from build123d import *

# Parameters (mm, degrees)
F0_W     = 274.2
F0_H     = 251.2
F1_DEPTH = 1
F3_DEPTH = 1.001
F4_R     = 1


with BuildPart() as f1:
    # F0 (on Top) → F1 (new body)
    with BuildSketch(Plane.XY):
        Rectangle(F0_W, F0_H)
    extrude(amount=F1_DEPTH)

    # F2 (on face) → F3 (cut, through all)
    with BuildSketch(Plane.XY.offset(1)):
        Polygon((-127.1, -66.8), (-127.1, -115.6), (-104.7, -115.6), (-104.7, -113.6), (-92.7, -113.6), (-92.7, -115.6), (-70.3, -115.6), (-70.3, -6), (-127.1, -6), (-127.1, -54.8), (-125.1, -54.8), (-125.1, -66.8), align=None)
        Polygon((-4.5, -6), (-61.3, -6), (-61.3, -54.8), (-59.3, -54.8), (-59.3, -66.8), (-61.3, -66.8), (-61.3, -115.6), (-38.9, -115.6), (-38.9, -113.6), (-26.9, -113.6), (-26.9, -115.6), (-4.5, -115.6), align=None)
        Polygon((61.3, -6), (4.5, -6), (4.5, -54.8), (6.5, -54.8), (6.5, -66.8), (4.5, -66.8), (4.5, -115.6), (26.9, -115.6), (26.9, -113.6), (38.9, -113.6), (38.9, -115.6), (61.3, -115.6), align=None)
        Polygon((127.1, -6), (70.3, -6), (70.3, -54.8), (72.3, -54.8), (72.3, -66.8), (70.3, -66.8), (70.3, -115.6), (92.7, -115.6), (92.7, -113.6), (104.7, -113.6), (104.7, -115.6), (127.1, -115.6), align=None)
        Polygon((127.1, 115.6), (70.3, 115.6), (70.3, 66.8), (72.3, 66.8), (72.3, 54.8), (70.3, 54.8), (70.3, 6), (92.7, 6), (92.7, 8), (104.7, 8), (104.7, 6), (127.1, 6), align=None)
        Polygon((61.3, 115.6), (4.5, 115.6), (4.5, 66.8), (6.5, 66.8), (6.5, 54.8), (4.5, 54.8), (4.5, 6), (26.9, 6), (26.9, 8), (38.9, 8), (38.9, 6), (61.3, 6), align=None)
        Polygon((-4.5, 115.6), (-61.3, 115.6), (-61.3, 66.8), (-59.3, 66.8), (-59.3, 54.8), (-61.3, 54.8), (-61.3, 6), (-38.9, 6), (-38.9, 8), (-26.9, 8), (-26.9, 6), (-4.5, 6), align=None)
        Polygon((-70.3, 115.6), (-127.1, 115.6), (-127.1, 66.8), (-125.1, 66.8), (-125.1, 54.8), (-127.1, 54.8), (-127.1, 6), (-104.7, 6), (-104.7, 8), (-92.7, 8), (-92.7, 6), (-70.3, 6), align=None)
    extrude(amount=-F3_DEPTH, mode=Mode.SUBTRACT)

    # F4
    f4_edges = [f1.edges().sort_by_distance(p)[0] for p in [
        (-127.1, -115.6, 0.5),
        (-104.7, -115.6, 0.5),
        (-92.7, -115.6, 0.5),
        (-70.3, -115.6, 0.5),
        (-70.3, -6, 0.5),
        (-127.1, -6, 0.5),
        (-127.1, -54.8, 0.5),
        (-127.1, -66.8, 0.5),
        (-61.3, -6, 0.5),
        (-4.5, -6, 0.5),
        (-61.3, -54.8, 0.5),
        (-61.3, -66.8, 0.5),
        (-61.3, -115.6, 0.5),
        (-38.9, -115.6, 0.5),
        (-26.9, -115.6, 0.5),
        (-4.5, -115.6, 0.5),
        (4.5, -115.6, 0.5),
        (26.9, -115.6, 0.5),
        (38.9, -115.6, 0.5),
        (61.3, -115.6, 0.5),
        (61.3, -6, 0.5),
        (4.5, -6, 0.5),
        (4.5, -54.8, 0.5),
        (4.5, -66.8, 0.5),
        (70.3, -6, 0.5),
        (70.3, -54.8, 0.5),
        (70.3, -66.8, 0.5),
        (70.3, -115.6, 0.5),
        (92.7, -115.6, 0.5),
        (104.7, -115.6, 0.5),
        (127.1, -115.6, 0.5),
        (127.1, -6, 0.5),
        (-127.1, 6, 0.5),
        (-104.7, 6, 0.5),
        (-92.7, 6, 0.5),
        (-70.3, 6, 0.5),
        (-70.3, 115.6, 0.5),
        (-127.1, 115.6, 0.5),
        (-127.1, 66.8, 0.5),
        (-127.1, 54.8, 0.5),
        (-61.3, 115.6, 0.5),
        (-61.3, 66.8, 0.5),
        (-61.3, 54.8, 0.5),
        (-61.3, 6, 0.5),
        (-38.9, 6, 0.5),
        (-26.9, 6, 0.5),
        (-4.5, 6, 0.5),
        (-4.5, 115.6, 0.5),
        (4.5, 115.6, 0.5),
        (4.5, 66.8, 0.5),
        (4.5, 54.8, 0.5),
        (4.5, 6, 0.5),
        (26.9, 6, 0.5),
        (38.9, 6, 0.5),
        (61.3, 6, 0.5),
        (61.3, 115.6, 0.5),
        (70.3, 115.6, 0.5),
        (70.3, 66.8, 0.5),
        (70.3, 54.8, 0.5),
        (70.3, 6, 0.5),
        (92.7, 6, 0.5),
        (104.7, 6, 0.5),
        (127.1, 6, 0.5),
        (127.1, 115.6, 0.5),
    ]]
    fillet(f4_edges, radius=F4_R)


solid = f1.part
Work out the finished part from the listing and answer in its coordinate system (mm). Give positions to 0.01 mm unless a question says otherwise; leave off trailing zeros. Loops run counter-clockwise (first coordinate to the right, second up) from the corner with the lowest first, then second, coordinate; pieces in that order, holes last. Notation, with made-up numbers: (-16, -13.5) - (3, -13.5) arc R25 cw to (3, -0.5) - close; hole circle Ø10 at (-38, -12.5). An arc over 180 degrees is marked (long way). Answer in a Markdown table with one row per item.
(1) Section C-C (y = -62) is taken. Give the vertices of the cut face in (x, z), and give its area (3 significant figures).
Results list:
| item | result |
|---|---|
| outline | (-137.1, 0) - (-125.1, 0) - (-125.1, 1) - (-137.1, 1) - close; (-70.3, 0) - (-59.3, 0) - (-59.3, 1) - (-70.3, 1) - close; (-4.5, 0) - (6.5, 0) - (6.5, 1) - (-4.5, 1) - close; (61.3, 0) - (72.3, 0) - (72.3, 1) - (61.3, 1) - close; (127.1, 0) - (137.1, 0) - (137.1, 1) - (127.1, 1) - close |
| area | 55.0 mm² |
(2) Section B-B (x = -81.5) is taken. Give the vertices of the cut face in (y, z), and give its area (3 significant figures).
Results list:
| item | result |
|---|---|
| outline | (-125.6, 0) - (-115.6, 0) - (-115.6, 1) - (-125.6, 1) - close; (-6, 0) - (6, 0) - (6, 1) - (-6, 1) - close; (115.6, 0) - (125.6, 0) - (125.6, 1) - (115.6, 1) - close |
| area | 32.0 mm² |
(3) Section D-D (x = -35) is taken. Give the vertices of the cut face in (y, z).
Results list:
| item | result |
|---|---|
| outline | (-125.6, 0) - (-113.6, 0) - (-113.6, 1) - (-125.6, 1) - close; (-6, 0) - (8, 0) - (8, 1) - (-6, 1) - close; (115.6, 0) - (125.6, 0) - (125.6, 1) - (115.6, 1) - close |
(4) Section A-A (y = 45) is taken. Give the vertices of the cut face in (x, z).
Results list:
| item | result |
|---|---|
| outline | (-137.1, 0) - (-127.1, 0) - (-127.1, 1) - (-137.1, 1) - close; (-70.3, 0) - (-61.3, 0) - (-61.3, 1) - (-70.3, 1) - close; (-4.5, 0) - (4.5, 0) - (4.5, 1) - (-4.5, 1) - close; (61.3, 0) - (70.3, 0) - (70.3, 1) - (61.3, 1) - close; (127.1, 0) - (137.1, 0) - (137.1, 1) - (127.1, 1) - close |
(5) Consider L1, parallel to Y at x = -118, z = 0.7; L2, parallel to X at y = 14, z = 0.4; L3, parallel to Y at x = -33, z = 0.65. Determine where each line is inside the solid, lowest interval first. Write a range as [from, to].
Results list:
| item | result |
|---|---|
| L1 | y = [-125.6, -115.6], [-6, 6], [115.6, 125.6] |
| L2 | x = [-137.1, -127.1], [-70.3, -61.3], [-4.5, 4.5], [61.3, 70.3], [127.1, 137.1] |
| L3 | y = [-125.6, -113.6], [-6, 8], [115.6, 125.6] |
